Read the model definition and answer for the solid it produces. Units are mm, in the model's axes. A direction names the side the tool comes from. Give positions to 0.01 mm unless a question says otherwise; leave off trailing zeros. Order: outer loops, then holes, each group sorted by start corner. A loop starts at its lowest first (then second) coordinate and runs counter-clockwise, first axis right, second up. Notation, with made-up numbers: (-22.75, 44.25) - (28.25, 44.25) arc R19 cw to (28.25, 54.25) - close; hole circle Ø7 at (83.5, 14.25). An arc over 180 degrees is marked (long way). Use a Markdown table: item, result. Add a question column.
1. A cutting plane is placed at B-B on z = 12.5. Determine the outline of the cut face in (x, y), and give its area (3 significant figures).
2. Consider L1, parallel to Y at x = 0, z = -5.25; L2, parallel to Y at x = 0, z = 6.4; L3, parallel to X at y = -5.5, z = 7. Determine where each line is inside the solid, lowest interval first.
3. For a pull along Z with two mould halves and no side action, classify faces 1 (the flat face through (0.1, -12.3, 25.45)), 2 (the cylindrical face through (-5.86, 11.267, 0.104)), 3 (the flat face through (-2.4, -1.2, 4.55)) as released by +Z, released by -Z, zero draft, split by the parting line, or undercut.
4. Which of the six approach directions +Z, -Z, +X, -X, +Y, -Y give full straight-line access (tool end or side, diameter ignored) to faces 4 (the flat face through (0, 0, 9.85)), 5 (the flat face through (6, 0, -15.15)), 6 (the conical face through (2.777, 12.507, -7.644))?
5. A cutting plane is placed at A-A on z = -3. Determine the outline of the cut face in (x, y), and give its area (3 significant figures).
6. A cutting plane is placed at C-C on z = 8. Determine the outline of the cut face in (x, y), and give its area (3 significant figures).
7. Flat-ended cylindrical pins translate along their axes: P1, Ø2.5, axis at x = -0.5, y = -0.5, coming from the -Z side; P2, Ø14.5, axis at x = 0, y = 0, coming from the +Z side; P3, Ø1.5, axis at x = 0.5, y = -5, coming from the +Z side. Find the tip coordinate at first contact, or state that the pin passes through.
```python
from build123d import *

# Parameters (mm, degrees)
SKETCH3_R          = 5.55
CUT_EXTRUDE1_DEPTH = 20
SKETCH4_R          = 2.4
CUT_EXTRUDE2_DEPTH = 25


with BuildPart() as part:
    # Sketch2 → Revolve1 (revolve)
    with BuildSketch(Plane(origin=(0, 0, 0), x_dir=(1, 0, 0), z_dir=(0, 1, 0)), mode=Mode.PRIVATE) as revolve1_sk:
        with BuildLine():
            Line((0, 15.45), (2, 15.45))
            Line((2, 15.45), (2, 15.15))
            Line((2, 15.15), (14.99, 15.15))
            Line((14.99, 15.15), (14.99, 11.45))
            Line((14.99, 11.45), (12.7, 7.45))
            Line((12.7, 7.45), (12.7, -7.45))
            Line((12.7, -7.45), (14.99, -11.45))
            Line((14.99, -11.45), (14.99, -15.15))
            Line((14.99, -15.15), (14.99, -25.45))
            Line((14.99, -25.45), (12, -25.45))
            add(Edge.make_bspline(
                [(0, -23.75), (6.057028237, -24.106745249), (12, -25.45)],
                knots=[0, 0, 0, 1, 1, 1], degree=2))
            Line((0, -23.75), (0, 0))
            Line((0, 0), (0, 15.45))
        make_face()
    revolve(revolve1_sk.sketch.rotate(Axis((0, 0, -30.524751378), (0, 0, 1)), 180), axis=Axis((0, 0, -30.524751378), (0, 0, 1)))

    # Sketch3 → Cut-Extrude1 (cut)
    with BuildSketch(Plane(origin=(0, 0, -15.45), x_dir=(-1, 0, 0), z_dir=(0, 0, -1))):
        Circle(SKETCH3_R)
    extrude(amount=-CUT_EXTRUDE1_DEPTH, mode=Mode.SUBTRACT)

    # Sketch4 → Cut-Extrude2 (cut)
    with BuildSketch(Plane(origin=(0, 0, -15.15), x_dir=(-1, 0, 0), z_dir=(0, 0, -1))):
        Circle(SKETCH4_R)
    extrude(amount=-CUT_EXTRUDE2_DEPTH, mode=Mode.SUBTRACT)


solid = part.part
```
Output values:
| question | item | result |
|---|---|---|
| 1 | outline | circle Ø29.98 at (0, 0) |
| 1 | area | 706 mm² |
| 2 | L1 | -12.7 to -5.55, 5.55 to 12.7 |
| 2 | L2 | -12.7 to -2.4, 2.4 to 12.7 |
| 2 | L3 | -11.45 to 11.45 |
| 3 | face 1 | released by +Z |
| 3 | face 2 | undercut |
| 3 | face 3 | released by -Z |
| 4 | face 4 | -Z |
| 4 | face 5 | -Z, +X, -X, +Y, -Y |
| 4 | face 6 | none |
| 5 | outline | circle Ø25.4 at (0, 0); hole circle Ø11.1 at (0, 0) |
| 5 | area | 410 mm² |
| 6 | outline | circle Ø26.03 at (0, 0); hole circle Ø4.8 at (0, 0) |
| 6 | area | 514 mm² |
| 7 | P1 | z = 9.85 |
| 7 | P2 | z = 24.54 |
| 7 | P3 | z = 24.32 |
